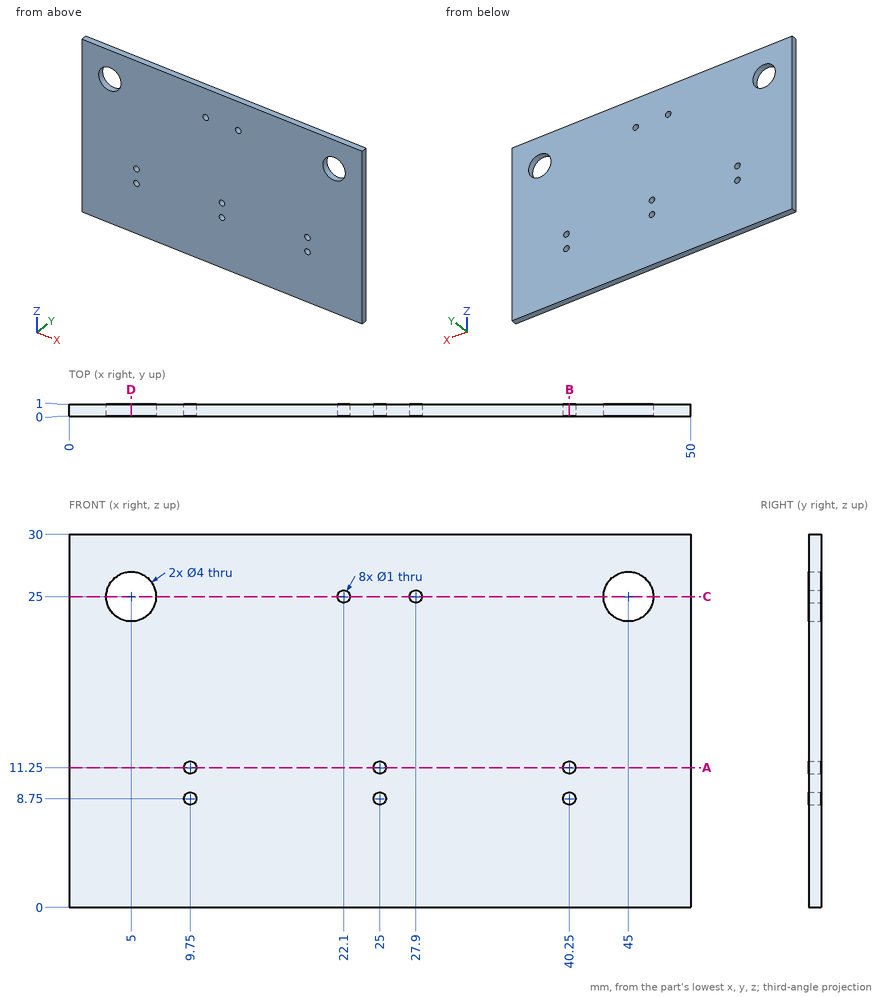
Verification items for this drawing (mm, ordinates from the low corner). Coordinates: 2 decimals unless noted, no trailing zeros. Write each loop counter-clockwise with the first axis right and the second up, starting at its lowest first coordinate (ties: lowest second). Pieces come first, ordered by that corner, then holes. Notation, with made-up numbers: (-33.75, 12.5) -> (-8.75, 12.5) arc R23 ccw to (-8.75, 20.5) -> close; hole circle Ø3 at (-11, 34.5). An arc over 180 degrees is marked (long way). One line per item, written item: value. Start each with the question number.
Q1. Cross-section at A-A on z = 11.25. Enter the section's corners in (x, y).
Q2. Go/stop test with a flat-tipped pin: P1, Ø3, axis at x = 5, z = 25, coming from the +Y side. Record where the tip stops, or that it passes through.
Q3. Cross-section at C-C on z = 25. Enter the section's corners in (x, y), and give its area (3 significant figures).
Q4. Thickness scan on L1, parallel to X at y = 0.75, z = 8.75; L2, parallel to Z at x = 9.75, y = 0.5; L3, parallel to X at y = 0.75, z = 25. Record the ranges inside material, lowest first. Write a range as from..to.
Q5. Cross-section at D-D on x = 5. Enter the section's corners in (y, z).
Q6. Cross-section at B-B on x = 40.25. Enter the section's corners in (y, z), and give its area (3 significant figures).
Checked values:
1. outline: (0, 0) -> (9.25, 0) -> (9.25, 1) -> (0, 1) -> close; (10.25, 0) -> (24.5, 0) -> (24.5, 1) -> (10.25, 1) -> close; (25.5, 0) -> (39.75, 0) -> (39.75, 1) -> (25.5, 1) -> close; (40.75, 0) -> (50, 0) -> (50, 1) -> (40.75, 1) -> close
2. P1: passes through
3. outline: (0, 0) -> (3, 0) -> (3, 1) -> (0, 1) -> close; (7, 0) -> (21.6, 0) -> (21.6, 1) -> (7, 1) -> close; (22.6, 0) -> (27.4, 0) -> (27.4, 1) -> (22.6, 1) -> close; (28.4, 0) -> (43, 0) -> (43, 1) -> (28.4, 1) -> close; (47, 0) -> (50, 0) -> (50, 1) -> (47, 1) -> close
3. area: 40.0 mm²
4. L1: x = 0..9.25, 10.25..24.5, 25.5..39.75, 40.75..50
4. L2: z = 0..8.25, 9.25..10.75, 11.75..30
4. L3: x = 0..3, 7..21.6, 22.6..27.4, 28.4..43, 47..50
5. outline: (0, 0) -> (1, 0) -> (1, 23) -> (0, 23) -> close; (0, 27) -> (1, 27) -> (1, 30) -> (0, 30) -> close
6. outline: (0, 0) -> (1, 0) -> (1, 8.25) -> (0, 8.25) -> close; (0, 9.25) -> (1, 9.25) -> (1, 10.75) -> (0, 10.75) -> close; (0, 11.75) -> (1, 11.75) -> (1, 30) -> (0, 30) -> close
6. area: 28.0 mm²
